Input: dimensioned drawing with shaded views. Units: mm. Origin: part minimum x, y, z. A direction names the side the tool comes from. Round coordinates to 2 decimals unless told otherwise and drop trailing zeros. Order: outer loops, then holes, each group sorted by start corner. A loop starts at its lowest first (then second) coordinate and runs counter-clockwise, first axis right, second up. Notation, with made-up numbers: M 53,84 L 59,84 A19 cw 59,119 Z; hole C 63.5,40.5 d11. An arc over 180 degrees is marked long. One line per question, with ' | ' between items.
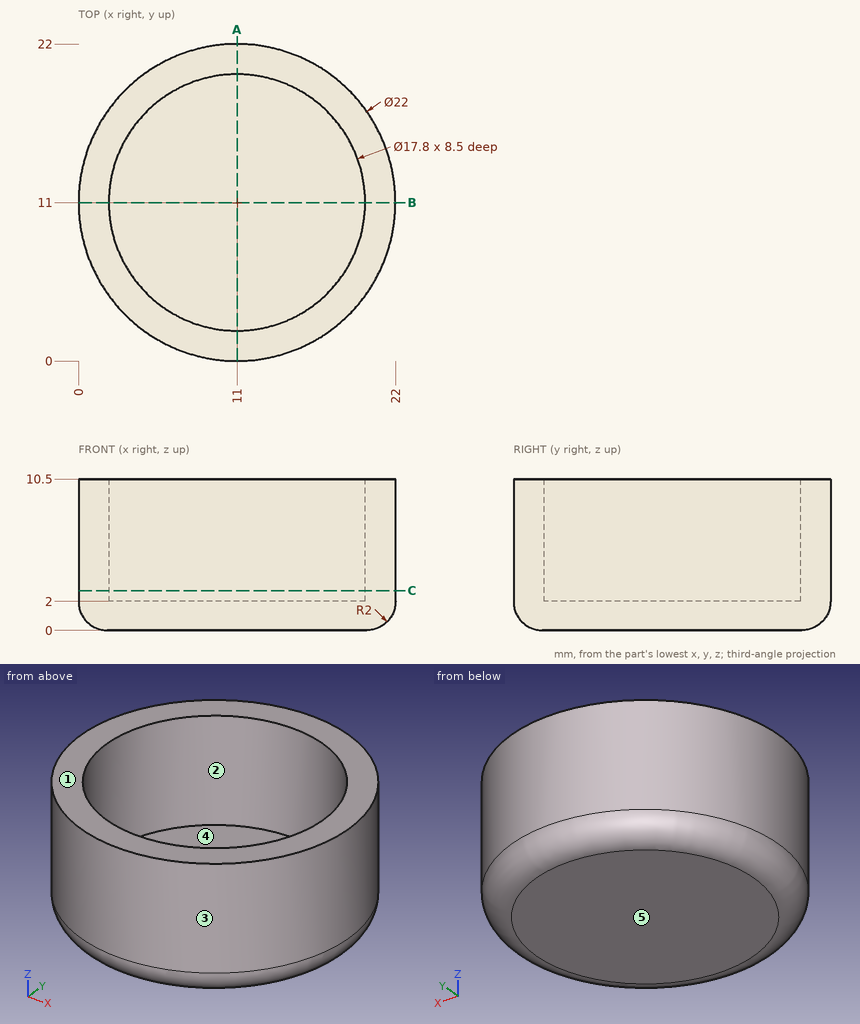
Item 1: First-contact query: pin 1 (6 mm diameter, centred on y = 7.5, z = 1.5, fed in from +X); pin 2 (3 mm diameter, centred on x = 6, z = 7, fed in from +Y); pin 3 (2 mm diameter, centred on x = 19.5, z = 5.5, fed in from +Y); pin 4 (4 mm diameter, centred on x = 19.5, y = 13.5, fed in from +Z). Flat tips, straight axial feed; report the tip coordinate or a pass-through.
Report:
pin 1: x = 21.99 | pin 2: y = 21.43 | pin 3: y = 19.05 | pin 4: z = 10.5
Item 2: Section query A-A, the plane x = 11. Return loops of the section in (y, z), plus the area to 3 significant figures.
Report:
outline: M 0,2 A2 ccw 2,0 L 20,0 A2 ccw 22,2 L 22,10.5 L 19.9,10.5 L 19.9,2 L 2.1,2 L 2.1,10.5 L 0,10.5 Z | area: 78.0 mm²
Item 3: Access query for the marked faces 1 and 2. Directions: +Z, -Z, +X, -X, +Y, -Y. A direction counts if a zero-diameter tool reaches every point of the face in a straight line with its end or side. Return the directions, or none.
Report:
face 1: +Z, +X, -X, +Y, -Y | face 2: +Z
Item 4: Section query C-C, the plane z = 2.75. Return loops of the section in (x, y), plus the area to 3 significant figures.
Report:
outline: C 11,11 d22; hole C 11,11 d17.8 | area: 131 mm²
Item 5: Line query: line 1 along Y through (x, z) = (11, 4.25); line 2 along Z through (x, y) = (8, 4.75). Output: solid intervals per line, ascending. Write a range as from..to.
Report:
line 1: 0..2.1, 19.9..22 | line 2: 0..2
Item 6: Mould query, pull axis X, two halves, no side actions, for the marked faces 3, 4 and 5. Classes: +X half, -X half, draft (parallel to the pull), parting line (faces both ways), or undercut.
Report:
face 3: parting line | face 4: undercut | face 5: draft
